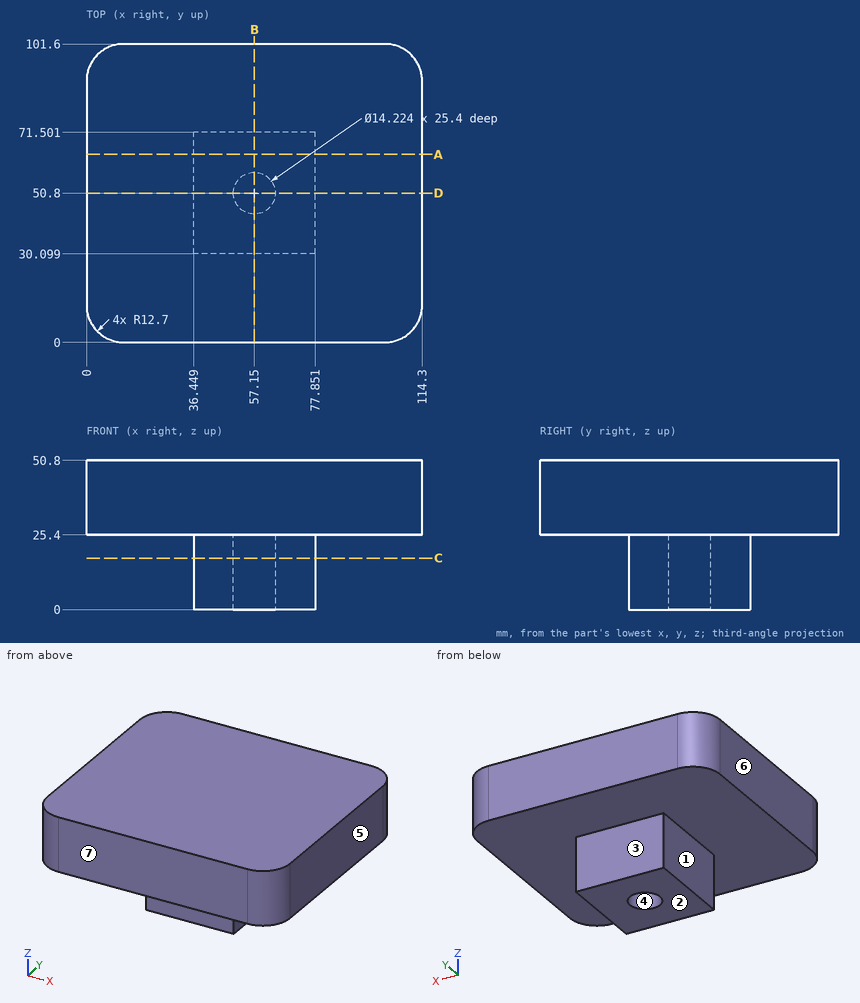
Geometry check sheet. Reference: drawing and pictorial views, mm from the part's lowest x, y, z. A direction names the side the tool comes from. Coordinates: 2 decimals unless noted, no trailing zeros. Order: outer loops, then holes, each group sorted by start corner. A loop starts at its lowest first (then second) coordinate and runs counter-clockwise, first axis right, second up. Notation, with made-up numbers: (22, -14.75) - (77, -14.75) arc R10 ccw to (77, 2.25) - close; hole circle Ø3 at (64.5, 58.25). An arc over 180 degrees is marked (long way). Answer in a Markdown table with one row per item. Add a question column.
1) Cross-section at B-B, the plane x = 57.15. Record the cut outline in (y, z), then the cut area to 3 significant figures.
2) Material ranges on line 1 along Y through (x, z) = (57.15, 9.5); line 2 along Z through (x, y) = (94, 46.5); line 3 along Y through (x, z) = (75, 17.5), recorded low to high. Write a range as [from, to].
3) Cross-section at A-A, the plane y = 64. Record the cut outline in (x, z), then the cut area to 3 significant figures.
4) Cross-section at D-D, the plane y = 50.8. Record the cut outline in (x, z).
5) Set-up check for the marked faces 1, 2 and 3: record each of +Z, -Z, +X, -X, +Y, -Y from which the full face is reachable in a straight line by a thin tool's end or side.
6) Cross-section at C-C, the plane z = 17.5. Record the cut outline in (x, y).
7) Release check for a two-part mould opening along X. For the marked faces 4, 5, 6 and 7 record: +X half, -X half, draft (parallel to the pull), parting line (faces both ways), or undercut.
8) Gauge pin test, flat ends, axial feed: P1, Ø7.5, axis at x = 48.5, z = 15, coming from the +Y side; P2, Ø10, axis at y = 52, z = 13, coming from the -X side; P3, Ø8.5, axis at x = 57.15, y = 50.8, coming from the -Z side. Record the tip position at first contact, or that the pin passes through.
Check result:
| question | item | result |
|---|---|---|
| 1 | outline | (0, 25.4) - (30.1, 25.4) - (30.1, 0) - (43.69, 0) - (43.69, 25.4) - (57.91, 25.4) - (57.91, 0) - (71.5, 0) - (71.5, 25.4) - (101.6, 25.4) - (101.6, 50.8) - (0, 50.8) - close |
| 1 | area | 3,270 mm² |
| 2 | line 1 | y = [30.1, 43.69], [57.91, 71.5] |
| 2 | line 2 | z = [25.4, 50.8] |
| 2 | line 3 | y = [30.1, 71.5] |
| 3 | outline | (0, 25.4) - (36.45, 25.4) - (36.45, 0) - (77.85, 0) - (77.85, 25.4) - (114.3, 25.4) - (114.3, 50.8) - (0, 50.8) - close |
| 3 | area | 3,950 mm² |
| 4 | outline | (0, 25.4) - (36.45, 25.4) - (36.45, 0) - (50.04, 0) - (50.04, 25.4) - (64.26, 25.4) - (64.26, 0) - (77.85, 0) - (77.85, 25.4) - (114.3, 25.4) - (114.3, 50.8) - (0, 50.8) - close |
| 5 | face 1 | -Z, -X, +Y, -Y |
| 5 | face 2 | -Z, +X, -X, +Y, -Y |
| 5 | face 3 | -Z, +X, -X, +Y |
| 6 | outline | (36.45, 30.1) - (77.85, 30.1) - (77.85, 71.5) - (36.45, 71.5) - close; hole circle Ø14.22 at (57.15, 50.8) |
| 7 | face 4 | undercut |
| 7 | face 5 | +X half |
| 7 | face 6 | -X half |
| 7 | face 7 | draft |
| 8 | P1 | stops at y = 71.5 |
| 8 | P2 | stops at x = 36.45 |
| 8 | P3 | stops at z = 25.4 |
